```python
from build123d import *

# Parameters (mm, degrees)
F1_R     = 38.1
F3_DEPTH = 19.05
F0_R     = 38.1
F4_DEPTH = 19.05
F2_R     = 38.1
F5_DEPTH = 38.1


with BuildPart() as f3:
    # F1 (on Top) → F3 (new body, symmetric)
    with BuildSketch(Plane.XY):
        Circle(F1_R)
    extrude(amount=F3_DEPTH, both=True)

    # F0 (on Front) → F4 (join, symmetric)
    with BuildSketch(Plane.XZ):
        Circle(F0_R)
    extrude(amount=F4_DEPTH, both=True)

    # F2 (on Right) → F5 (join)
    with BuildSketch(Plane.YZ):
        Circle(F2_R)
    extrude(amount=F5_DEPTH)


solid = f3.part
```
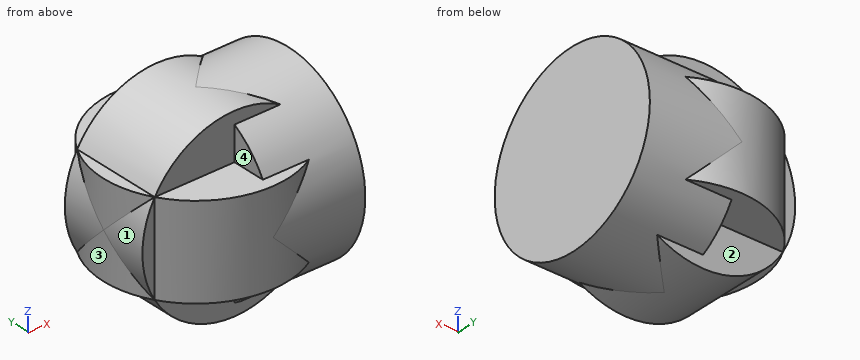
Verification items for the finished model (mm, model axes). Face numbers are marked on the shaded views. A direction names the side the tool comes from. Coordinates: 2 decimals unless noted, no trailing zeros. Order: outer loops, then holes, each group sorted by start corner. A loop starts at its lowest first (then second) coordinate and runs counter-clockwise, first axis right, second up. Notation, with made-up numbers: (-32.5, 29.5) - (-14.5, 29.5) arc R31 ccw to (-14.5, 66.5) - close; hole circle Ø9 at (81.5, 34.5). An arc over 180 degrees is marked (long way). Return JSON: item names as keys, results as strings.
(1) Section check C-C, the plane z = 21. Record the cut outline in (x, y).
Filled sheet:
{"outline": "(-31.79, -19.05) - (0, -19.05) - (0, -31.79) - (38.1, -31.79) - (38.1, 31.79) - (0, 31.79) - (0, 19.05) - (-31.79, 19.05) - close"}
(2) Section check B-B, the plane y = 28. Record the cut outline in (x, z), and give its area (3 significant figures).
Filled sheet:
{"outline": "(-25.84, -19.05) - (0, -19.05) - (0, -25.84) - (38.1, -25.84) - (38.1, 25.84) - (0, 25.84) - (0, 19.05) - (-25.84, 19.05) - close", "area": "2,950 mm^2"}
(3) Section check A-A, the plane x = 9. Record the cut outline in (y, z), and give its area (3 significant figures).
Filled sheet:
{"outline": "(-37.02, -19.05) - (-33, -19.05) arc R38.1 ccw to (-19.05, -33) - (-19.05, -37.02) - (-9, -37.02) arc R38.1 ccw to (9, -37.02) - (19.05, -37.02) - (19.05, -33) arc R38.1 ccw to (33, -19.05) - (37.02, -19.05) - (37.02, -9) arc R38.1 ccw to (37.02, 9) - (37.02, 19.05) - (33, 19.05) arc R38.1 ccw to (19.05, 33) - (19.05, 37.02) - (9, 37.02) arc R38.1 ccw to (-9, 37.02) - (-19.05, 37.02) - (-19.05, 33) arc R38.1 ccw to (-33, 19.05) - (-37.02, 19.05) - (-37.02, 9) arc R38.1 ccw to (-37.02, -9) - close", "area": "4,700 mm^2"}
(4) Go/stop test with flat-tipped pins: pin 1 (15.5 mm diameter, centred on y = 28, z = -23.5, fed in from -X); pin 2 (15 mm diameter, centred on x = 0, z = 28.5, fed in from +Y); pin 3 (4 mm diameter, centred on y = -27, z = 25.5, fed in from -X). Record where each tip stops, or that it passes through.
Filled sheet:
{"pin 1": "stops at x = -31.35", "pin 2": "stops at y = 31.79", "pin 3": "stops at x = 0"}
(5) Thickness scan on line 1 along Y through (x, z) = (-20.5, 28.5); line 2 along X through (y, z) = (33, -7.5). Record the ranges inside material, lowest first.
Filled sheet:
{"line 1": "y = -19.05 to 19.05", "line 2": "x = -19.04 to 38.1"}
(6) Section check D-D, the plane y = -11.5. Record the cut outline in (x, z), and give its area (3 significant figures).
Filled sheet:
{"outline": "(-36.32, -19.05) - (-33, -19.05) arc R38.1 ccw to (11.5, -36.32) - (38.1, -36.32) - (38.1, 36.32) - (11.5, 36.32) arc R38.1 ccw to (-33, 19.05) - (-36.32, 19.05) - (-36.32, 11.5) arc R38.1 ccw to (-36.32, -11.5) - close", "area": "5,100 mm^2"}
(7) Access from +Z, -Z, +X, -X, +Y, -Y to the whole of each face (thin tool, end or side, straight path). Record for the marked faces 1, 2, 3 and 4.
Filled sheet:
{"face 1": "-X, -Y", "face 2": "-Z, -X, +Y", "face 3": "-Z, -X", "face 4": "+Z, -X, -Y"}
